CAD build for the part. Positions are in the model's coordinates, mm. A direction names the side the tool comes from. Coordinates: 2 decimals unless noted, no trailing zeros. Loops run counter-clockwise (first coordinate to the right, second up) from the corner with the lowest first, then second, coordinate; pieces in that order, holes last. Notation, with made-up numbers: (9.25, 74) -> (55.25, 74) arc R28 ccw to (55.25, 107) -> close; hole circle Ø6 at (-37, 30.25). An arc over 180 degrees is marked (long way). Return JSON: item names as keys, results as strings. Group by question number.
(1) Saw through at C-C on y = 15.25. Write the cut outline in (x, z), then the cut area to 3 significant figures.
(2) Probe L1, parallel to X at y = 14.75, z = 0; L2, parallel to Y at x = -4.5, z = 8; L3, parallel to Y at x = 9, z = -2.5. List the from-to ranges inside material, lowest first.
(3) Saw through at B-B on x = 0. Write the cut outline in (y, z), then the cut area to 3 significant figures.
(4) Saw through at A-A on z = 0. Write the cut outline in (x, y).
(5) Mould opens along X. For faces 1 (the face through (-2.628, 13.148, -8.346)), 2 (the face through (-2, 0, 2)), 3 (the face through (-2.44, 11.09, -0.54)) say: pulls with the +X half, pulls with the -X half, needs draft (parallel to the pull), parting line crosses it, or undercut.
(6) Flat gauge pins, fed straight in: pin 1 Ø5 at (y, z) = (9, -2.5) entering from +X; pin 2 Ø10 at (y, z) = (9, 2.5) entering from +X; pin 3 Ø10 at (x, y) = (-6, 14.5) entering from -Z. Where does each tip first touch, or does it go through?
(7) Tool access for faces 4 (the face through (1.921, 20.625, -8.649)), 5 (the face through (-2, 22.5, 2)): list every direction of +Z, -Z, +X, -X, +Y, -Y with a clear straight run to the whole face (end or side of a thin tool).
```python
from build123d import *

# Parameters (mm, degrees)
SKETCH1_R           = 12
SKETCH1_R_2         = 2.5
BOSS_EXTRUDE1_DEPTH = 6
SKETCH2_R           = 8.750000000000002
SKETCH2_R_2         = 2.5
BOSS_EXTRUDE2_DEPTH = 14.5
SKETCH3_R           = 10.5
SKETCH3_R_2         = 2.5
BOSS_EXTRUDE3_DEPTH = 2


with BuildPart() as part:
    # Sketch1 → Boss-Extrude1 (new body)
    with BuildSketch(Plane(origin=(0, 0, 0), x_dir=(1, 0, 0), z_dir=(0, 1, 0))):
        with Locations(Location((0, 0, 0), (0, 0, 270))):
            Circle(SKETCH1_R)
        with Locations(Location((0, 0, 0), (0, 0, 270))):
            Circle(SKETCH1_R_2, mode=Mode.SUBTRACT)
    extrude(amount=BOSS_EXTRUDE1_DEPTH)

    # Sketch2 → Boss-Extrude2 (add)
    with BuildSketch(Plane(origin=(0, 6, 0), x_dir=(1, 0, 0), z_dir=(0, 1, 0))):
        with Locations(Location((0, 0, 0), (0, 0, 90))):
            Circle(SKETCH2_R)
        with Locations(Location((0, 0, 0), (0, 0, 270))):
            Circle(SKETCH2_R_2, mode=Mode.SUBTRACT)
    extrude(amount=BOSS_EXTRUDE2_DEPTH)

    # Sketch3 → Boss-Extrude3 (add)
    with BuildSketch(Plane(origin=(0, 20.5, 0), x_dir=(1, 0, 0), z_dir=(0, 1, 0))):
        with Locations(Location((0, 0, 0), (0, 0, 270))):
            Circle(SKETCH3_R)
        with Locations(Location((0, 0, 0), (0, 0, 270))):
            Circle(SKETCH3_R_2, mode=Mode.SUBTRACT)
    extrude(amount=BOSS_EXTRUDE3_DEPTH)

    # Cut-Sweep3: sweep along a curve in space
    with BuildLine() as cut_sweep3_path:
        ThreePointArc((0, 20.5, 8.750000000000002), (6.187184335382292, 20.5, 6.187184335382293), (8.750000000000002, 20.5, 0))
        ThreePointArc((8.750000000000002, 20.5, 0), (6.187184335382293, 20.5, -6.187184335382292), (0, 20.5, -8.750000000000002))
        ThreePointArc((0, 20.5, -8.750000000000002), (-6.187184335382292, 20.5, -6.187184335382293), (-8.750000000000002, 20.5, 0))
        ThreePointArc((-8.750000000000002, 20.5, 0), (-6.187184335382293, 20.5, 6.187184335382292), (0, 20.5, 8.750000000000002))
    # Sketch5 → Cut-Sweep3 (sweep, cut)
    with BuildSketch(Plane.XY):
        Polygon((-10.5, 22.5), (-8.750000000000002, 20.5), (-10.5, 20.5), align=None)
    sweep(path=cut_sweep3_path.line, mode=Mode.SUBTRACT)

    # Cut-Sweep4: sweep along a curve in space
    with BuildLine() as cut_sweep4_path:
        ThreePointArc((0, 6, 12.000000000000002), (8.485281374238571, 6, 8.485281374238571), (12.000000000000002, 6, 0))
        ThreePointArc((12.000000000000002, 6, 0), (8.485281374238571, 6, -8.485281374238571), (0, 6, -12.000000000000002))
        ThreePointArc((0, 6, -12.000000000000002), (-8.485281374238571, 6, -8.485281374238571), (-12.000000000000002, 6, 0))
        ThreePointArc((-12.000000000000002, 6, 0), (-8.485281374238571, 6, 8.485281374238571), (0, 6, 12.000000000000002))
    # Sketch6 → Cut-Sweep4 (sweep, cut)
    with BuildSketch(Plane.XY):
        with BuildLine():
            Line((-12.000000000000002, 3), (-12.000000000000002, 6))
            Line((-12.000000000000002, 6), (-9.000000000000002, 6.000000000000002))
            ThreePointArc((-9.000000000000002, 6.000000000000002), (-11.121320343559645, 5.121320343559644), (-12.000000000000002, 3))
        make_face()
    sweep(path=cut_sweep4_path.line, mode=Mode.SUBTRACT)

    # Cut-Sweep5: sweep along a curve in space
    with BuildLine() as cut_sweep5_path:
        ThreePointArc((0, 0, 12.000000000000002), (8.485281374238571, 0, 8.485281374238571), (12.000000000000002, 0, 0))
        ThreePointArc((12.000000000000002, 0, 0), (8.485281374238571, 0, -8.485281374238571), (0, 0, -12.000000000000002))
        ThreePointArc((0, 0, -12.000000000000002), (-8.485281374238571, 0, -8.485281374238571), (-12.000000000000002, 0, 0))
        ThreePointArc((-12.000000000000002, 0, 0), (-8.485281374238571, 0, 8.485281374238571), (0, 0, 12.000000000000002))
    # Sketch7 → Cut-Sweep5 (sweep, cut)
    with BuildSketch(Plane.XY):
        with BuildLine():
            Line((-9.000000000000002, -1.3e-15), (-12.000000000000002, 0))
            Line((-12.000000000000002, 0), (-12.000000000000002, 2.999999999999979))
            ThreePointArc((-12.000000000000002, 2.999999999999979), (-11.121320343559637, 0.8786796564403496), (-9.000000000000002, -1.3e-15))
        make_face()
    sweep(path=cut_sweep5_path.line, mode=Mode.SUBTRACT)


solid = part.part
```
Geometry results:
{
 "1": {"outline": "circle Ø17.5 at (0, 0); hole circle Ø5 at (0, 0)", "area": "221 mm²"},
 "2": {"L1": "-8.75 to -2.5, 2.5 to 8.75", "L2": "0.01 to 5.99, 20.99 to 22.5", "L3": "0.02 to 5.98, 21.18 to 22.5"},
 "3": {"outline": "(0, -9) arc R3 ccw to (6, -9) -> (6, -8.75) -> (20.5, -8.75) -> (22.5, -10.5) -> (22.5, -2.5) -> (0, -2.5) -> close; (0, 2.5) -> (22.5, 2.5) -> (22.5, 10.5) -> (20.5, 8.75) -> (6, 8.75) -> (6, 9) arc R3 ccw to (0, 9) -> close", "area": "316 mm²"},
 "4": {"outline": "(-10.5, 22.5) -> (-8.75, 20.5) -> (-8.75, 6) -> (-9, 6) arc R3 ccw to (-9, 0) -> (-2.5, 0) -> (-2.5, 22.5) -> close; (2.5, 0) -> (9, 0) arc R3 ccw to (9, 6) -> (8.75, 6) -> (8.75, 20.5) -> (10.5, 22.5) -> (2.5, 22.5) -> close"},
 "5": {"face 1": "parting line crosses it", "face 2": "needs draft", "face 3": "undercut"},
 "6": {"pin 1": "x = 8.75", "pin 2": "x = 11.7", "pin 3": "z = -8.69"},
 "7": {"face 4": "none", "face 5": "+Z, -Z, +X, -X, +Y"}
}
